Autodesk Fusion 360 part; units mm, degrees
sketch "Sketch1" plane through (0, 0, 0) normal (0, 1, 0) x (1, 0, 0)
  line L0 (0, 0) -> (52, 0)
  line L1 (52, 0) -> (52, -10)
  line L2 (52, -10) -> (0, -10)
  line L3 (0, -10) -> (0, 0)
  line L4 (0, 0) -> (5, 0)
  line L5 (5, 0) -> (5, 10)
  line L6 (5, 10) -> (0, 10)
  line L7 (0, 10) -> (0, 0)
  dimension "d1" = 52
  dimension "d2" = 10
  dimension "d3" = 5
  dimension "d4" = 10
extrude "Extrude1" add sketch "Sketch1" along normal blind 45
sketch "Sketch2" plane through (0, 45, 0) normal (0, 1, 0) x (-1, 0, 0)
  line L0 (-5, 0) -> (-5, -10)
  line L1 (-5, -10) -> (0, -10)
  line L2 (0, -10) -> (0, 10)
  line L3 (0, 10) -> (-52, 10)
  line L4 (-52, 10) -> (-52, 0)
  line L5 (-52, 0) -> (-5, 0)
  line L6 (-49, 7.834) -> (-42.269, 7.834)
  line L7 (-42.269, 7.834) -> (-42.269, 5.174)
  line L8 (-42.269, 5.174) -> (-49, 5.174)
  line L9 (-49, 5.174) -> (-49, 7.834)
  line L10 (-49, 7.834) -> (-42.269, 5.174) construction
  line L11 (-42.269, 7.834) -> (-49, 5.174) construction
  line L12 (-47.7345, 10) -> (-43.5345, 10)
  line L13 (-43.5345, 10) -> (-43.5345, 9)
  line L14 (-43.5345, 9) -> (-47.7345, 9)
  line L15 (-47.7345, 9) -> (-47.7345, 10)
  line L16 (-47.7345, 10) -> (-43.5345, 9) construction
  line L17 (-43.5345, 10) -> (-47.7345, 9) construction
  line L18 (-47.7345, 9) -> (-49, 7.834)
  line L19 (-43.5345, 9) -> (-42.269, 7.834)
  line L20 (-45.6345, 6.504) -> (-45.6345, 9.5)
  point P0 (-45.6345, 6.504)
  point P1 (-45.6345, 9.5)
  dimension "rail_upper_part_depth" = 1
  dimension "rail_upper_part_width" = 4.2
  dimension "rail_depth" = 4.826
  dimension "rail_base_depth" = 2.66
  dimension "rail_edge_position" = 3
  dimension "rail_base_width" = 6.731
extrude "Extrude2" cut sketch "Sketch2" against normal up to surface (45 mm away) contours L3 L12 L13 L14 L15 | L6 L14 L18 L20 | L6 L14 L19 L20 | L6 L7 L8 L9
ref_plane "WorkPlane1" through (36.8045, 22.5, 9.5) normal (1, 0, 0) x (0, 0, 1)
sketch "Sketch3" plane through (36.8045, 22.5, 9.5) normal (1, 0, 0) x (0, 0, -1)
  line L0 (-0.5, -22.5) -> (-15.5, -22.5)
  line L1 (-15.5, -22.5) -> (-15.5, 22.5)
  line L2 (-15.5, 22.5) -> (-0.5, 22.5)
  line L3 (-0.5, 22.5) -> (-0.5, -22.5)
  line L4 (-0.5, 22.5) -> (9.5, 22.5)
  line L5 (9.5, -22.5) -> (-0.5, -22.5)
  line L6 (-0.5, -22.5) -> (-0.5, 22.5)
  line L7 (-15.5, -15.25) -> (-4, -15.25)
  line L8 (-4, -15.25) -> (-4, 15.25)
  line L9 (-4, 15.25) -> (-15.5, 15.25)
  line L10 (-15.5, 15.25) -> (-15.5, -15.25)
  line L11 (-15.5, -15.25) -> (-4, 15.25) construction
  line L12 (-4, -15.25) -> (-15.5, 15.25) construction
  circle A0 centre (-10.5, -18.5) radius 1.5
  line L13 (-15.5, 0) -> (-4, 0)
  circle A1 centre (-10.5, 18.5) radius 1.5
  point P0 (-9.75, 0)
  dimension "moto_holder_frae_length" = 15
  dimension "motor_width_space" = 30.5
  dimension "d22" = 22.5
  dimension "d23" = 37
  dimension "d25" = 3
  dimension "holes_from_surface2" = 10
  dimension "d27" = 3.5
extrude "Extrude3" add sketch "Sketch3" against normal blind 5 contours L0 L1 L2 L3 L6 L7 L8 L9
sketch "Sketch4" plane through (5, 0, 0) normal (1, 0, 0) x (0, 0, -1)
  line L0 (0, 0) -> (10, 0)
  line L1 (10, 0) -> (10, 45)
  line L2 (10, 45) -> (0, 45)
  line L3 (0, 45) -> (0, 0)
  line L4 (10, 22.5) -> (0, 22.5)
  circle A0 centre (5, 37.5) radius 1.5
  circle A1 centre (5, 7.5) radius 1.5
  dimension "d30" = 3
  dimension "d31" = 5
  dimension "d32" = 30
extrude "Extrude4" cut sketch "Sketch4" against normal up to surface (5 mm away) contours A0 | A1
equation "d22 = d5 / 2"
Geometry check sheet. Reference: the model listing, model coordinates, mm. A direction names the side the tool comes from. Coordinates: 2 decimals unless noted, no trailing zeros. Loops run counter-clockwise (first coordinate to the right, second up) from the corner with the lowest first, then second, coordinate; pieces in that order, holes last.
Item 1: Access from +Z, -Z, +X, -X, +Y, -Y to the whole of each face (thin tool, end or side, straight path). Record for faces 1 (the face through (42.269, 23, 7)), 2 (the face through (31.804, 28, 13)), 3 (the face through (28, 22, 0)), 4 (the face through (36.804, 28, 13)), 5 (the face through (34, 7.25, 19)).
Item 2: Sectioned sample at B-B, the plane y = 4. Record the boundary of the cut face in (x, z), then the cut area to 3 significant figures.
Item 3: Thickness scan on line 1 (Y direction, x = 1, z = -5); line 2 (Y direction, x = 34, z = 20); line 3 (X direction, y = 41, z = 5.5). Record the ranges inside material, lowest first.
Item 4: Release check for a two-part mould opening along Y. For faces 6 (the face through (16, 22, 10)), 7 (the face through (2.54, 6.17, -5.69)), 8 (the face through (24, 45, 5)) record: released by +Y, released by -Y, zero draft, split by the parting line, or undercut.
Item 5: Go/stop test with flat-tipped pins: pin 1 Ø3.5 at (x, y) = (40, 24.5) entering from +Z; pin 2 Ø2.5 at (x, y) = (35, 21) entering from +Z; pin 3 Ø1.5 at (x, y) = (45, 15.5) entering from -Z. Record where each tip stops, or that it passes through.
Item 6: Sectioned sample at C-C, the plane z = 17.5. Record the boundary of the cut face in (x, y).
Item 7: Sectioned sample at A-A, the plane z = -5. Record the boundary of the cut face in (x, y).
Item 8: Sectioned sample at D-D, the plane x = 3. Record the boundary of the cut face in (y, z), then the cut area to 3 significant figures.
Check result:
1. face 1: +Y, -Y
1. face 2: +Z, -X, +Y, -Y
1. face 3: -Z, +X, +Y, -Y
1. face 4: +Z, +X, +Y, -Y
1. face 5: +Z, +X, -X
2. outline: (0, -10) - (5, -10) - (5, 0) - (52, 0) - (52, 10) - (47.73, 10) - (47.73, 9) - (49, 7.83) - (49, 5.17) - (42.27, 5.17) - (42.27, 7.83) - (43.53, 9) - (43.53, 10) - (36.8, 10) - (36.8, 18.5) - (31.8, 18.5) - (31.8, 10) - (0, 10) - close; (31.8, 21.5) - (36.8, 21.5) - (36.8, 25) - (31.8, 25) - close
2. area: 602 mm2
3. line 1: y = 0 to 6, 9 to 36, 39 to 45
3. line 2: y = 0 to 2.5, 5.5 to 7.25, 37.75 to 39.5, 42.5 to 45
3. line 3: x = 0 to 42.27, 49 to 52
4. face 6: zero draft
4. face 7: undercut
4. face 8: released by +Y
5. pin 1: stops at z = 10
5. pin 2: stops at z = 13.5
5. pin 3: stops at z = 0
6. outline: (31.8, 0) - (36.8, 0) - (36.8, 7.25) - (31.8, 7.25) - close; (31.8, 37.75) - (36.8, 37.75) - (36.8, 45) - (31.8, 45) - close
7. outline: (0, 0) - (5, 0) - (5, 6) - (0, 6) - close; (0, 9) - (5, 9) - (5, 36) - (0, 36) - close; (0, 39) - (5, 39) - (5, 45) - (0, 45) - close
8. outline: (0, -10) - (45, -10) - (45, 10) - (0, 10) - close; hole circle Ø3 at (7.5, -5); hole circle Ø3 at (37.5, -5)
8. area: 886 mm2
